Part model, mm, in its own coordinate system. Face numbers are marked on the shaded views. Give positions to 0.01 mm unless a question says otherwise; leave off trailing zeros. Write each loop counter-clockwise with the first axis right and the second up, starting at its lowest first coordinate (ties: lowest second). Pieces come first, ordered by that corner, then holes. Notation, with made-up numbers: M 17,-19 L 53,-19 A21 ccw 53,-1 Z; hole C -39.5,83 d3. An arc over 180 degrees is marked long. Answer as CSV lines item,"result". Start each with the question number.
Item 1: Wall check: L1, parallel to Y at x = 0, z = 7.25; L2, parallel to Z at x = -2.5, y = -3; L3, parallel to Z at x = 0.25, y = -1.5. Give the ranges that are in metal, low to high. Write a range as from..to.
Item 2: Band-saw the part on A-A, the plane y = 0. List the corners of the cut face in (x, z).
Item 3: Two-plate mould, pull along X, no slides. Class the marked faces 1, 2 and 3: +X half, -X half, draft (parallel to the pull), parting line (faces both ways), or undercut.
Item 4: Band-saw the part on D-D, the plane z = -1. List the corners of the cut face in (x, y).
Item 5: Band-saw the part on C-C, the plane z = 12.5. List the corners of the cut face in (x, y), then the cut area to 3 significant figures.
Item 6: Pin check, flat tips, straight feed: pin 1 (3 mm diameter, centred on y = 1, z = -1, fed in from +X); pin 2 (1 mm diameter, centred on x = 0.5, y = 1.5, fed in from -Z); pin 3 (1.5 mm diameter, centred on y = -1.5, z = 4.5, fed in from +X); pin 4 (4 mm diameter, centred on y = 0.5, z = 3.5, fed in from -X). Stop position of each tip, or through.
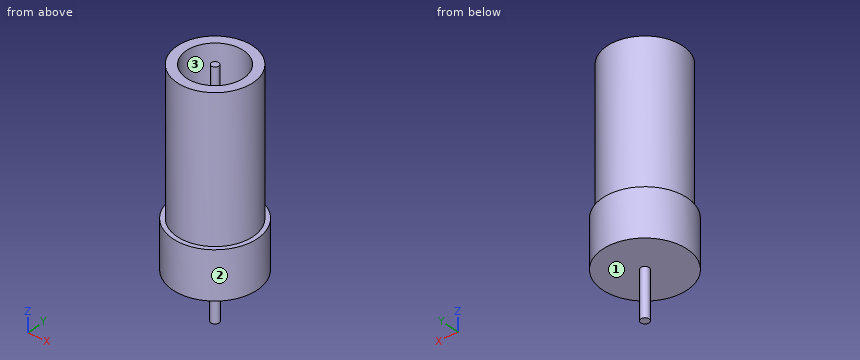
from build123d import *

# Parameters (mm, degrees)
SKETCH1_R           = 4
SKETCH1_R_2         = 3
BOSS_EXTRUDE1_DEPTH = 15
SKETCH2_R           = 3
BOSS_EXTRUDE3_DEPTH = 15
SKETCH3_R           = 3.009782436
SKETCH3_R_2         = 0.386251133
CUT_EXTRUDE2_DEPTH  = 13
SKETCH4_R           = 4.454105624
BOSS_EXTRUDE4_DEPTH = 5
SKETCH5_R           = 0.442435296
BOSS_EXTRUDE5_DEPTH = 5


with BuildPart() as part:
    # Sketch1 → Boss-Extrude1 (new body)
    with BuildSketch(Plane.XY):
        Circle(SKETCH1_R)
        Circle(SKETCH1_R_2, mode=Mode.SUBTRACT)
    extrude(amount=BOSS_EXTRUDE1_DEPTH)

    # Sketch2 → Boss-Extrude3 (add)
    with BuildSketch(Plane(origin=(0, 0, 0), x_dir=(-1, 0, 0), z_dir=(0, 0, -1))):
        Circle(SKETCH2_R)
    extrude(amount=-BOSS_EXTRUDE3_DEPTH)

    # Sketch3 → Cut-Extrude2 (cut)
    with BuildSketch(Plane.XY.offset(15)):
        Circle(SKETCH3_R)
        Circle(SKETCH3_R_2, mode=Mode.SUBTRACT)
    extrude(amount=-CUT_EXTRUDE2_DEPTH, mode=Mode.SUBTRACT)

    # Sketch4 → Boss-Extrude4 (add)
    with BuildSketch(Plane(origin=(0, 0, 0), x_dir=(-1, 0, 0), z_dir=(0, 0, -1))):
        Circle(SKETCH4_R)
    extrude(amount=BOSS_EXTRUDE4_DEPTH)

    # Sketch5 → Boss-Extrude5 (add)
    with BuildSketch(Plane(origin=(0, 0, -5), x_dir=(-1, 0, 0), z_dir=(0, 0, -1))):
        Circle(SKETCH5_R)
    extrude(amount=BOSS_EXTRUDE5_DEPTH)


solid = part.part
Output:
1,L1,"-4..-3.01, -0.39..0.39, 3.01..4"
1,L2,"-5..15"
1,L3,"-5..2"
2,outline,"M -4.45,-5 L -0.44,-5 L -0.44,-10 L 0.44,-10 L 0.44,-5 L 4.45,-5 L 4.45,0 L 4,0 L 4,15 L 3.01,15 L 3.01,2 L 0.39,2 L 0.39,15 L -0.39,15 L -0.39,2 L -3.01,2 L -3.01,15 L -4,15 L -4,0 L -4.45,0 Z"
3,face 1,"draft"
3,face 2,"parting line"
3,face 3,"undercut"
4,outline,"C 0,0 d8.91"
5,outline,"C 0,0 d8; C 0,0 d0.77; hole C 0,0 d6.02"
5,area,"22.3 mm²"
6,pin 1,"x = 4.45"
6,pin 2,"z = -5"
6,pin 3,"x = 3.93"
6,pin 4,"x = -4"
